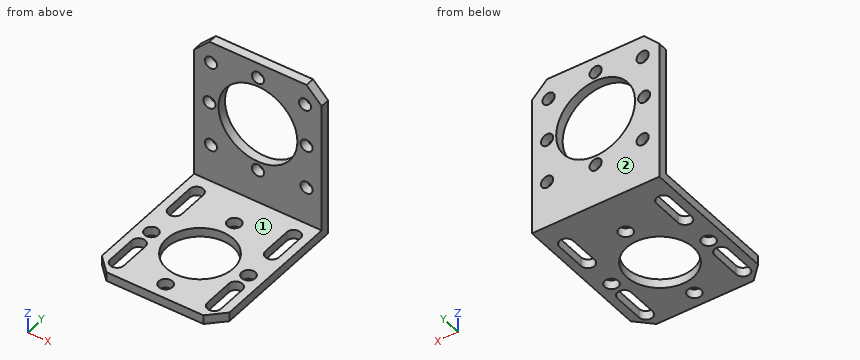
```python
from build123d import *

# Parameters (mm, degrees)
SKETCH_1_W          = 42
SKETCH_1_H          = 51
EXTRUDE_1_DEPTH     = 3
SKETCH_2_W          = 42
SKETCH_2_H          = 3
EXTRUDE_2_DEPTH     = 48
CHAMFER_1_SIZE      = 5
SKETCH_3_R          = 13
SKETCH_3_R_2        = 2
CUT_EXTRUDE_1_DEPTH = 48
SKETCH_4_R          = 2.25
SKETCH_4_R_2        = 11
CUT_EXTRUDE_2_DEPTH = 48


with BuildPart() as part:
    # 스케치1 → 보스-돌출1 (new body)
    with BuildSketch(Plane.XY):
        Rectangle(SKETCH_1_W, SKETCH_1_H)
    extrude(amount=EXTRUDE_1_DEPTH)

    # 스케치2 → 보스-돌출2 (add)
    with BuildSketch(Plane.XY.offset(3)):
        with Locations((0, 24)):
            Rectangle(SKETCH_2_W, SKETCH_2_H)
    extrude(amount=EXTRUDE_2_DEPTH)

    # 모따기1
    chamfer_1_edges = [part.edges().sort_by_distance(p)[0] for p in [
        (-21, 24, 51),
        (21, 24, 51),
        (21, -25.5, 1.5),
        (-21, -25.5, 1.5),
    ]]
    chamfer(chamfer_1_edges, length=CHAMFER_1_SIZE)

    # 스케치3 → 컷-돌출1 (cut)
    with BuildSketch(Plane.XZ.offset(-22.5)):
        with Locations((0, 30)):
            Circle(SKETCH_3_R)
        with Locations((-15.5, 44)):
            Circle(SKETCH_3_R_2)
        with Locations((-15.5, 15.5)):
            Circle(SKETCH_3_R_2)
        with Locations((0, 46)):
            Circle(SKETCH_3_R_2)
        with Locations((15.5, 44)):
            Circle(SKETCH_3_R_2)
        with Locations((16, 30)):
            Circle(SKETCH_3_R_2)
        with Locations((0, 14)):
            Circle(SKETCH_3_R_2)
        with Locations((-16, 30)):
            Circle(SKETCH_3_R_2)
        with Locations((16, 15.5)):
            Circle(SKETCH_3_R_2)
    extrude(amount=-CUT_EXTRUDE_1_DEPTH, mode=Mode.SUBTRACT)

    # 스케치4 → 컷-돌출2 (cut)
    with BuildSketch(Plane.XY.offset(3)):
        with Locations((0, -20.5)):
            Circle(SKETCH_4_R)
        with Locations((0, -4.5)):
            Circle(SKETCH_4_R_2)
        with Locations((-16, -4.5)):
            Circle(SKETCH_4_R)
        with Locations((0, 11.5)):
            Circle(SKETCH_4_R)
        with Locations((16, -4.5)):
            Circle(SKETCH_4_R)
        with BuildLine():
            Line((-13.75, 16.5), (-13.75, 6.5))
            ThreePointArc((-13.75, 6.5), (-16, 4.25), (-18.25, 6.5))
            Line((-18.25, 6.5), (-18.25, 16.5))
            ThreePointArc((-18.25, 16.5), (-16, 18.75), (-13.75, 16.5))
        make_face()
        with BuildLine():
            Line((-13.75, -10.5), (-13.75, -20.5))
            ThreePointArc((-13.75, -20.5), (-16, -22.75), (-18.25, -20.5))
            Line((-18.25, -20.5), (-18.25, -10.5))
            ThreePointArc((-18.25, -10.5), (-16, -8.25), (-13.75, -10.5))
        make_face()
        with BuildLine():
            Line((13.75, -10.5), (13.75, -20.5))
            ThreePointArc((13.75, -20.5), (16, -22.75), (18.25, -20.5))
            Line((18.25, -20.5), (18.25, -10.5))
            ThreePointArc((18.25, -10.5), (16, -8.25), (13.75, -10.5))
        make_face()
        with BuildLine():
            Line((13.75, 16.5), (13.75, 6.5))
            ThreePointArc((13.75, 6.5), (16, 4.25), (18.25, 6.5))
            Line((18.25, 6.5), (18.25, 16.5))
            ThreePointArc((18.25, 16.5), (16, 18.75), (13.75, 16.5))
        make_face()
    extrude(amount=-CUT_EXTRUDE_2_DEPTH, mode=Mode.SUBTRACT)


solid = part.part
```
Work out the finished part from the listing and answer in its coordinate system (mm). Face numbers are marked on the shaded views. A direction names the side the tool comes from. Give positions to 0.01 mm unless a question says otherwise; leave off trailing zeros. Order: outer loops, then holes, each group sorted by start corner. A loop starts at its lowest first (then second) coordinate and runs counter-clockwise, first axis right, second up. Notation, with made-up numbers: (-31, -40) -> (15, -40) arc R17 cw to (15, -19) -> close; hole circle Ø10 at (-21.75, -5.5). An arc over 180 degrees is marked (long way). Answer as CSV lines item,"result". Start each with the question number.
(1) Section A-A, the plane y = 15 is taken. Write down the section's boundary in (x, z), plus the area to 3 significant figures.
(2) Which of the six approach directions +Z, -Z, +X, -X, +Y, -Y give full straight-line access (tool end or side, diameter ignored) to the marked faces 1 and 2?
(3) Section D-D, the plane x = -5 is taken. Write down the section's boundary in (y, z), plus the area to 3 significant figures.
(4) Section C-C, the plane z = 30 is taken. Write down the section's boundary in (x, y), plus the area to 3 significant figures.
(5) Each of these flat-tipped pins is pushed along its axis until it touches: pin 1 Ø7 at (x, y) = (16, -4.5) entering from +Z; pin 2 Ø4 at (x, z) = (-8.5, 19) entering from -Y. Where does it stop, or does it pass through?
(6) Section B-B, the plane x = 0 is taken. Give the number of separate pieces and of enclosed holes in the cut face, plus the area to 3 significant figures.
(7) Consider line 1 along Y through (x, z) = (0, 2.1); line 2 along Y through (x, z) = (16, 0.7); line 3 along Z through (x, y) = (-16, 24.95). Determine where each line is inside the solid, lowest interval first.
Entries:
1,outline,"(-21, 0) -> (-18.25, 0) -> (-18.25, 3) -> (-21, 3) -> close; (-13.75, 0) -> (13.75, 0) -> (13.75, 3) -> (-13.75, 3) -> close; (18.25, 0) -> (21, 0) -> (21, 3) -> (18.25, 3) -> close"
1,area,"99.0 mm²"
2,face 1,"+Z, +X, -X, -Y"
2,face 2,"+Z, -Z, +X, -X, +Y"
3,outline,"(-25.5, 0) -> (-14.3, 0) -> (-14.3, 3) -> (-25.5, 3) -> close; (5.3, 0) -> (25.5, 0) -> (25.5, 18) -> (22.5, 18) -> (22.5, 3) -> (5.3, 3) -> close; (22.5, 42) -> (25.5, 42) -> (25.5, 51) -> (22.5, 51) -> close"
3,area,"166 mm²"
4,outline,"(-21, 22.5) -> (-18, 22.5) -> (-18, 25.5) -> (-21, 25.5) -> close; (-14, 22.5) -> (-13, 22.5) -> (-13, 25.5) -> (-14, 25.5) -> close; (13, 22.5) -> (14, 22.5) -> (14, 25.5) -> (13, 25.5) -> close; (18, 22.5) -> (21, 22.5) -> (21, 25.5) -> (18, 25.5) -> close"
4,area,"24.0 mm²"
5,pin 1,"z = 3"
5,pin 2,"y = 22.5"
6,separate pieces,"7"
6,enclosed holes,"0"
6,area,"102 mm²"
7,line 1,"-25.5 to -22.75, -18.25 to -15.5, 6.5 to 9.25, 13.75 to 25.5"
7,line 2,"-25.5 to -22.75, -8.25 to -6.75, -2.25 to 4.25, 18.75 to 25.5"
7,line 3,"0 to 13.56, 17.44 to 28, 32 to 42.06, 45.94 to 51"
